For this review, take the finished solid that the model builds, in its own axes (mm). Face numbers are marked on the shaded views. A direction names the side the tool comes from. Round coordinates to 2 decimals unless told otherwise and drop trailing zeros. Order: outer loops, then holes, each group sorted by start corner. A loop starts at its lowest first (then second) coordinate and runs counter-clockwise, first axis right, second up. Notation, with made-up numbers: (26, -5.5) -> (76, -5.5) arc R19 ccw to (76, 30.5) -> close; hole circle Ø4 at (26.5, 53). An arc over 180 degrees is marked (long way). Answer in a Markdown table with one row per item.
```python
from build123d import *

# Parameters (mm, degrees)
BOSS_EXTRUDE1_DEPTH     = 13
CUT_EXTRUDE1_DEPTH      = 10
CUT_EXTRUDE1_DEPTH_BACK = 30
SKETCH2_R               = 1.6
SKETCH2_R_2             = 1.611537585
SKETCH3_R               = 3
CUT_EXTRUDE2_DEPTH      = 1
SKETCH4_R               = 2.9
CUT_EXTRUDE3_DEPTH      = 1
CHAMFER1_SIZE           = 10
FILLET1_R               = 4


with BuildPart() as part:
    # Sketch1 → Boss-Extrude1 (new body)
    with BuildSketch(Plane.XY.offset(98.171636097)):
        Polygon((30.334370899, 78.263460463), (35.214370899, 78.263460463), (35.214370899, 65.863460463), (35.214370899, 63.263460463), (25.584370899, 63.263460463), (25.584370899, 49.763460463), (22.584370899, 49.763460463), (22.584370899, 63.263460463), (22.584370899, 63.763460463), (30.334370899, 63.763460463), align=None)
    extrude(amount=-BOSS_EXTRUDE1_DEPTH)

    # Sketch2 → Cut-Extrude1 (cut, two sides: drawn at the far end of the back side and taken through both)
    with BuildSketch(Plane(origin=(35.214370899, 0, 0), x_dir=(0, 0, -1), z_dir=(1, 0, 0)).offset(-CUT_EXTRUDE1_DEPTH_BACK)):
        with Locations(Location((-91.671636097, 75.863460463, 0), (0, 0, 180))):
            Circle(SKETCH2_R)
        with Locations(Location((-91.671636097, 54.263460463, 0), (0, 0, 180))):
            Circle(SKETCH2_R_2)
    extrude(amount=CUT_EXTRUDE1_DEPTH + CUT_EXTRUDE1_DEPTH_BACK, mode=Mode.SUBTRACT)

    # Sketch3 → Cut-Extrude2 (cut)
    with BuildSketch(Plane.ZY.offset(-22.584370899)):
        with Locations((91.671636097, 54.263460463)):
            Circle(SKETCH3_R)
    extrude(amount=-CUT_EXTRUDE2_DEPTH, mode=Mode.SUBTRACT)

    # Sketch4 → Cut-Extrude3 (cut)
    with BuildSketch(Plane.ZY.offset(-30.334370899)):
        with Locations((91.671636097, 75.863460463)):
            Circle(SKETCH4_R)
    extrude(amount=-CUT_EXTRUDE3_DEPTH, mode=Mode.SUBTRACT)

    # Chamfer1
    # the kernel refuses this chamfer: 10 mm, written as the material it adds along each edge
    with BuildSketch(Plane(origin=(30.334370899, 63.763460463, 98.171636097), x_dir=(0.027495876610586337, 0.9996219169112968, 0), z_dir=(0, 0, -1))) as chamfer1_piece_1_section:
        Polygon((CHAMFER1_SIZE * 0.999621916911, -CHAMFER1_SIZE * 0.0274958766106), (-CHAMFER1_SIZE * 0.0274958766106, -CHAMFER1_SIZE * 0.999621916911), (0, 0), align=None)
    chamfer1_piece_1 = extrude(amount=13, mode=Mode.PRIVATE)
    chamfer1_piece_1 = chamfer1_piece_1 - Plane(origin=(27.388550815, 75.863460463, 91.671636097), x_dir=(0, 0, 1), z_dir=(-1, 0, 0)) * Cylinder(2.9, 66, mode=Mode.PRIVATE)
    chamfer1_piece_1 = split(chamfer1_piece_1, bisect_by=Plane(origin=(22.584370899, 67.23157259, 91.671636099), z_dir=(1, 0, 0)), keep=Keep.TOP, mode=Mode.PRIVATE)
    add(chamfer1_piece_1)

    # Fillet1
    fillet1_edges = [part.edges().sort_by_distance(p)[0] for p in [
        (24.084370899, 49.763460463, 98.171636097),
    ]]
    fillet(fillet1_edges, radius=FILLET1_R)


solid = part.part
```
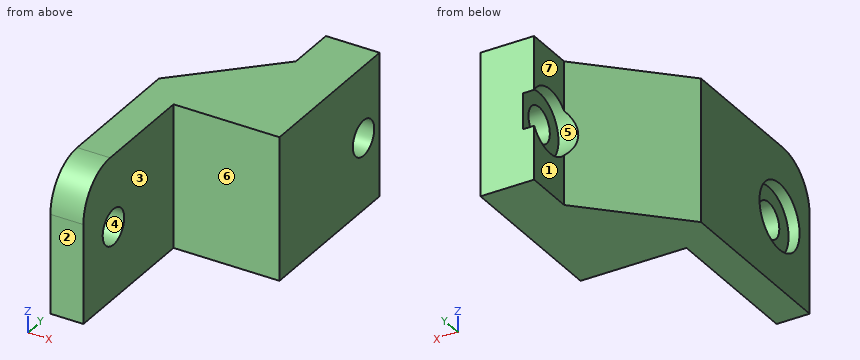
Q1. Clearance check with flat-ended pins moving along their axes: pin 1 Ø5 at (y, z) = (55, 89.5) entering from -X; pin 2 Ø2 at (x, z) = (29, 87) entering from +Y; pin 3 Ø3.5 at (y, z) = (54.26, 91.67) entering from -X; pin 4 Ø6 at (y, z) = (75, 92.5) entering from -X. State where each tip first meets the part, or that it passes through.
Answer key:
| item | result |
|---|---|
| pin 1 | stops at x = 22.58 |
| pin 2 | stops at y = 73.43 |
| pin 3 | stops at x = 23.58 |
| pin 4 | stops at x = 28.57 |
Q2. The part is to be moulded in two halves that separate along Y. For the marked faces 4, 5, 6 and 7, say which applies: +Y half, -Y half, draft (parallel to the pull), parting line (faces both ways), or undercut.
Answer key:
| item | result |
|---|---|
| face 4 | undercut |
| face 5 | undercut |
| face 6 | -Y half |
| face 7 | draft |
Q3. To check wall thickness, follow probe 1 along Y at (x, z) = (31.5, 91.75); probe 2 along X at (y, z) = (59.25, 89.75); probe 3 along Y at (x, z) = (33, 93). State the ranges of each line that lie inside material, in increasing order.
Answer key:
| item | result |
|---|---|
| probe 1 | y = 63.26 to 74.27, 77.46 to 78.26 |
| probe 2 | x = 22.58 to 25.58 |
| probe 3 | y = 63.26 to 74.97, 76.76 to 78.26 |
Q4. Take a section at C-C, the plane y = 52. Write out the cut boundary in (x, z), then the cut area to 3 significant figures.
Answer key:
| item | result |
|---|---|
| outline | (22.58, 85.17) -> (25.58, 85.17) -> (25.58, 97.76) -> (22.58, 97.76) -> (22.58, 93.64) -> (23.58, 93.64) -> (23.58, 89.7) -> (22.58, 89.7) -> close |
| area | 33.8 mm^2 |
Q5. Take a section at B-B, the plane x = 32.25. Write out the cut boundary in (y, z).
Answer key:
| item | result |
|---|---|
| outline | (63.26, 85.17) -> (78.26, 85.17) -> (78.26, 98.17) -> (63.26, 98.17) -> close; hole circle Ø3.2 at (75.86, 91.67) |
Q6. Take a section at A-A, the plane z = 93. Write out the cut boundary in (x, y).
Answer key:
| item | result |
|---|---|
| outline | (22.58, 49.76) -> (25.58, 49.76) -> (25.58, 53.35) -> (23.58, 53.35) -> (23.58, 51.57) -> (22.58, 51.57) -> close; (22.58, 56.95) -> (23.58, 56.95) -> (23.58, 55.18) -> (25.58, 55.18) -> (25.58, 63.26) -> (35.21, 63.26) -> (35.21, 74.97) -> (31.33, 74.97) -> (31.33, 73.29) -> (29.86, 73.29) -> (22.58, 66.01) -> close; (31.33, 76.76) -> (35.21, 76.76) -> (35.21, 78.26) -> (31.33, 78.26) -> close |
Q7. Tool access review of the marked faces 1, 2 and 3: name each direction out of +Z, -Z, +X, -X, +Y, -Y from which nothing blocks a thin tool from reaching the whole face with its end or side.
Answer key:
| item | result |
|---|---|
| face 1 | +Z, -Z, -X, +Y |
| face 2 | +Z, -Z, +X, -X, -Y |
| face 3 | +Z, -Z, +X, -Y |
Q8. Take a section at D-D, the plane z = 91.5. Write out the cut boundary in (x, y), then the cut area to 3 significant figures.
Answer key:
| item | result |
|---|---|
| outline | (22.58, 49.76) -> (25.58, 49.76) -> (25.58, 52.66) -> (23.58, 52.66) -> (23.58, 51.27) -> (22.58, 51.27) -> close; (22.58, 57.26) -> (23.58, 57.26) -> (23.58, 55.87) -> (25.58, 55.87) -> (25.58, 63.26) -> (35.21, 63.26) -> (35.21, 74.27) -> (31.33, 74.27) -> (31.33, 72.97) -> (29.54, 72.97) -> (22.58, 66.01) -> close; (31.33, 77.45) -> (35.21, 77.45) -> (35.21, 78.26) -> (31.33, 78.26) -> close |
| area | 135 mm^2 |
